Input: part model. Units: mm. Frame: model coordinates. Give positions to 0.01 mm unless a question says otherwise; leave off trailing zeros. Loops run counter-clockwise (first coordinate to the right, second up) from the corner with the lowest first, then second, coordinate; pieces in that order, holes last. Notation, with made-up numbers: (66.25, -22.75) - (70.25, -22.75) arc R29 cw to (70.25, 4.25) - close; hole circle Ø8 at (16, 36.25). An arc over 180 degrees is marked (long way). Answer as a JSON object with one key per item and string values. Group by question number.
(1) Pin query (flat end, axial travel): P1, Ø5, axis at x = 12.7, z = 6.35, coming from the -Y side; P2, Ø5, axis at y = -6, z = 2, coming from the +X side. Return the tip coordinate at first contact, or that it passes through.
(2) Material intervals for L1, parallel to Z at x = 12.7, y = -17.7; L2, parallel to Z at x = 12.7, y = -8.25 (3 decimals); L3, parallel to X at y = -17.25, z = 8, sorted ascending.
(3) Section query D-D (z = 2). Return loops of the section in (x, y), plus the area to 3 significant figures.
(4) Section query C-C (z = 6.35). Return loops of the section in (x, y) (3 decimals).
(5) Section query B-B (y = -6). Return loops of the section in (x, z) (3 decimals), plus the area to 3 significant figures.
(6) Section query A-A (x = 12.7). Return loops of the section in (y, z) (3 decimals), plus the area to 3 significant figures.
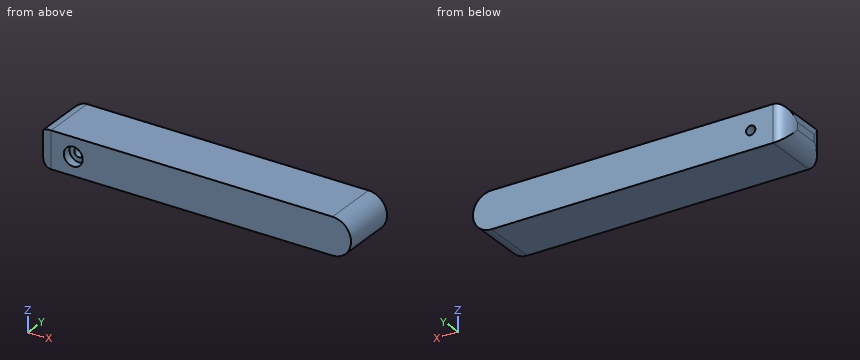
```python
from build123d import *

# Parameters (mm, degrees)
F1_DEPTH       = 19.05
F2_R           = 5.08
F4_D           = 3.15
F4_CBORE_D     = 6.5
F4_CBORE_DEPTH = 3


with BuildPart() as f1:
    # F0 (on Front) → F1 (new body)
    with BuildSketch(Plane.XZ):
        with BuildLine():
            Line((0, 12.7), (0, 0))
            Line((0, 0), (101.6, 0))
            ThreePointArc((101.6, 0), (107.95, 6.35), (101.6, 12.7))
            Line((101.6, 12.7), (0, 12.7))
        make_face()
    extrude(amount=F1_DEPTH)

    # F2
    f2_edges = [f1.edges().sort_by_distance(p)[0] for p in [
        (0, -19.05, 6.35),
        (0, -9.525, 12.7),
        (0, 0, 6.35),
        (0, -9.525, 0),
    ]]
    fillet(f2_edges, radius=F2_R)

    # F4 (through all)
    with Locations(Plane.XZ.offset(19.05)):
        with Locations((12.7, 6.35)):
            CounterBoreHole(F4_D / 2, F4_CBORE_D / 2, F4_CBORE_DEPTH)


solid = f1.part
```
Recorded:
{
 "1": {"P1": "stops at y = -16.05", "P2": "stops at x = 107.67"},
 "2": {"L1": "z = 0 to 3.1, 9.6 to 12.7", "L2": "z = 0 to 4.775, 7.925 to 12.7", "L3": "x = 1.2 to 9.9, 15.5 to 107.73"},
 "3": {"outline": "(1.04, -17.05) arc R5.08 ccw to (5.08, -19.05) - (106.23, -19.05) - (106.23, 0) - (5.08, 0) arc R5.08 ccw to (1.04, -2) - close", "area": "2,000 mm^2"},
 "4": {"outline": "(0, -13.97) arc R5.08 ccw to (5.08, -19.05) - (9.45, -19.05) - (9.45, -16.05) - (11.125, -16.05) - (11.125, 0) - (5.08, 0) arc R5.08 ccw to (0, -5.08) - close; (14.275, -16.05) - (15.95, -16.05) - (15.95, -19.05) - (107.95, -19.05) - (107.95, 0) - (14.275, 0) - close"},
 "5": {"outline": "(0, 5.08) arc R5.08 ccw to (5.08, 0) - (101.6, 0) arc R6.35 ccw to (101.6, 12.7) - (5.08, 12.7) arc R5.08 ccw to (0, 7.62) - close; hole circle Ø3.15 at (12.7, 6.35)", "area": "1,330 mm^2"},
 "6": {"outline": "(-19.05, 0) - (0, 0) - (0, 4.775) - (-16.05, 4.775) - (-16.05, 3.1) - (-19.05, 3.1) - close; (-19.05, 9.6) - (-16.05, 9.6) - (-16.05, 7.925) - (0, 7.925) - (0, 12.7) - (-19.05, 12.7) - close", "area": "172 mm^2"}
}
